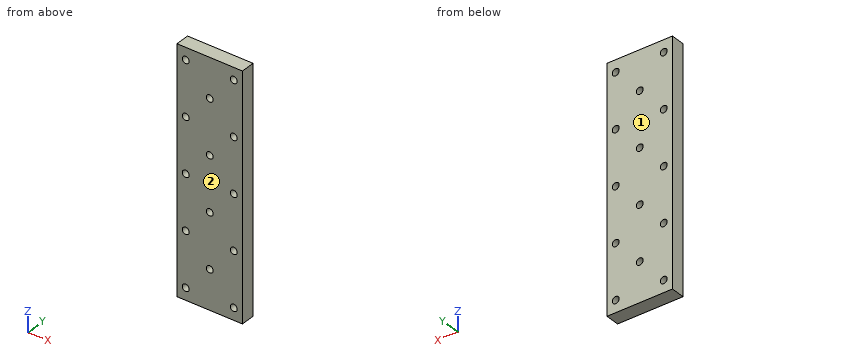
Autodesk Inventor part; units mm, degrees
ref_plane "YZ Plane" through (0, 0, 0) normal (1, 0, 0) x (0, 1, 0)
ref_plane "XZ Plane" through (0, 0, 0) normal (0, 1, 0) x (-1, 0, 0)
ref_plane "XY Plane" through (0, 0, 0) normal (0, 0, 1) x (1, 0, 0)
sketch "Sketch1" plane through (0, 0, 0) normal (0, 1, 0) x (-1, 0, 0)
  circle A0 centre (0, 0) radius 10.45 construction
  circle A1 centre (0, 0) radius 1.5875
  circle A2 centre (0, -25) radius 9.9 construction
  circle A3 centre (0, -25) radius 1.5875
  circle A4 centre (0, -50) radius 9.57 construction
  circle A5 centre (0, -50) radius 1.5875
  circle A6 centre (0, -75) radius 9.35 construction
  circle A7 centre (0, -75) radius 1.5875
  line L0 (15, 18) -> (-15, 18)
  line L1 (-15, 18) -> (-15, -93)
  line L2 (-15, -93) -> (15, -93)
  line L3 (15, -93) -> (15, 18)
  circle A8 centre (0, 0) radius 11.45 construction
  circle A9 centre (0, -25) radius 10.9 construction
  circle A10 centre (0, -50) radius 10.57 construction
  circle A11 centre (0, -75) radius 10.35 construction
  circle A12 centre (11, -12.5) radius 1.5875
  line L4 (0, 0) -> (0, -25) construction
  line L5 (0, 0) -> (-15, 0) construction
  line L6 (0, -25) -> (-15, -25) construction
  line L7 (0, -50) -> (-15, -50) construction
  line L8 (0, -75) -> (-15, -75) construction
  circle A13 centre (-11, -12.5) radius 1.5875
  circle A14 centre (11, 12.5) radius 1.5875
  circle A15 centre (-11, 12.5) radius 1.5875
  circle A16 centre (11, -37.5) radius 1.5875
  circle A17 centre (-11, -37.5) radius 1.5875
  circle A18 centre (11, -62.5) radius 1.5875
  circle A19 centre (-11, -62.5) radius 1.5875
  circle A20 centre (11, -87.5) radius 1.5875
  circle A21 centre (-11, -87.5) radius 1.5875
  point P0 (0, -12.5)
  dimension "d0" = 20.9
  dimension "d1" = 3.175
  dimension "d2" = 19.8
  dimension "d3" = 3.175
  dimension "d4" = 19.14
  dimension "d5" = 3.175
  dimension "d6" = 18.7
  dimension "d7" = 3.175
  dimension "d8" = 25
  dimension "d9" = 25
  dimension "d10" = 25
  dimension "d11" = 15
  dimension "d12" = 15
  dimension "d13" = 18
  dimension "d14" = 18
  dimension "d15" = 1
  dimension "d16" = 1
  dimension "d17" = 1
  dimension "d18" = 1
  dimension "d19" = 3.175
  dimension "d20" = 4
extrude "Extrusion2" add sketch "Sketch1" along normal blind 6.39
equation "\"d23\" = WoodThickness"
properties part number "BearingSilicone_Base"
Work out the finished part from the listing and answer in its coordinate system (mm). Face numbers are marked on the shaded views. Give positions to 0.01 mm unless a question says otherwise; leave off trailing zeros. Order: outer loops, then holes, each group sorted by start corner. A loop starts at its lowest first (then second) coordinate and runs counter-clockwise, first axis right, second up. Notation, with made-up numbers: M 45.5,-18 L 60.5,-18 A15 cw 60.5,-1 Z; hole C -12.5,-17 d9. An arc over 180 degrees is marked long. Return JSON: item names as keys, results as strings.
1) Section A-A, the plane x = 0 is taken. Write down the section's boundary in (y, z), plus the area to 3 significant figures.
Resolved:
{"outline": "M 0,-93 L 6.39,-93 L 6.39,-76.59 L 0,-76.59 Z; M 0,-73.41 L 6.39,-73.41 L 6.39,-51.59 L 0,-51.59 Z; M 0,-48.41 L 6.39,-48.41 L 6.39,-26.59 L 0,-26.59 Z; M 0,-23.41 L 6.39,-23.41 L 6.39,-1.59 L 0,-1.59 Z; M 0,1.59 L 6.39,1.59 L 6.39,18 L 0,18 Z", "area": "628 mm^2"}
2) Straight lines are drawn through the part: line 1 along Z through (x, y) = (0, 3.5); line 2 along Z through (x, y) = (-10.75, 3.25); line 3 along X through (y, z) = (5, -87.5). For each, find the intervals that lie inside material, in ascending order. Write a range as [from, to].
Resolved:
{"line 1": "[-93, -76.59], [-73.41, -51.59], [-48.41, -26.59], [-23.41, -1.59], [1.59, 18]", "line 2": "[-93, -89.07], [-85.93, -64.07], [-60.93, -39.07], [-35.93, -14.07], [-10.93, 10.93], [14.07, 18]", "line 3": "[-15, -12.59], [-9.41, 9.41], [12.59, 15]"}
3) Section C-C, the plane x = 11 is taken. Write down the section's boundary in (y, z), plus the area to 3 significant figures.
Resolved:
{"outline": "M 0,-93 L 6.39,-93 L 6.39,-89.09 L 0,-89.09 Z; M 0,-85.91 L 6.39,-85.91 L 6.39,-64.09 L 0,-64.09 Z; M 0,-60.91 L 6.39,-60.91 L 6.39,-39.09 L 0,-39.09 Z; M 0,-35.91 L 6.39,-35.91 L 6.39,-14.09 L 0,-14.09 Z; M 0,-10.91 L 6.39,-10.91 L 6.39,10.91 L 0,10.91 Z; M 0,14.09 L 6.39,14.09 L 6.39,18 L 0,18 Z", "area": "608 mm^2"}
4) Section D-D, the plane y = 4.75 is taken. Give the number of separate pieces and of enclosed holes in the cut face, plus the area to 3 significant figures.
Resolved:
{"separate pieces": "1", "enclosed holes": "14", "area": "3,220 mm^2"}
5) Section B-B, the plane z = -62.5 is taken. Write down the section's boundary in (x, y).
Resolved:
{"outline": "M -15,0 L -12.59,0 L -12.59,6.39 L -15,6.39 Z; M -9.41,0 L 9.41,0 L 9.41,6.39 L -9.41,6.39 Z; M 12.59,0 L 15,0 L 15,6.39 L 12.59,6.39 Z"}
6) For a pull along Y with two mould halves and no side action, classify the marked faces 1 and 2 as +Y half, -Y half, draft (parallel to the pull), parting line (faces both ways), or undercut.
Resolved:
{"face 1": "+Y half", "face 2": "-Y half"}
